```python
from build123d import *

# Parameters (mm, degrees)
EXTRUDE_START                = -12
EXTRUDE_1_DEPTH              = 12
HOLE_WIZARD_M5_1_D           = 4.2
HOLE_WIZARD_M5_1_DEPTH       = 12.4
HOLE_WIZARD_M5_1_CBORE_D     = 5
HOLE_WIZARD_M5_1_CBORE_DEPTH = 10
HOLE_WIZARD_M5_1_TIP         = 1.2618073
HOLE_WIZARD_M5_2_D           = 4.2
HOLE_WIZARD_M5_2_DEPTH       = 12.4
HOLE_WIZARD_M5_2_CBORE_D     = 5
HOLE_WIZARD_M5_2_CBORE_DEPTH = 10
HOLE_WIZARD_M5_2_TIP         = 1.2618073
HOLE_WIZARD_M5_3_D           = 4.2
HOLE_WIZARD_M5_3_DEPTH       = 12.4
HOLE_WIZARD_M5_3_CBORE_D     = 5
HOLE_WIZARD_M5_3_CBORE_DEPTH = 10
HOLE_WIZARD_M5_3_TIP         = 1.2618073
HOLE_WIZARD_M5_4_D           = 4.2
HOLE_WIZARD_M5_4_DEPTH       = 12.4
HOLE_WIZARD_M5_4_CBORE_D     = 5
HOLE_WIZARD_M5_4_CBORE_DEPTH = 10
HOLE_WIZARD_M5_4_TIP         = 1.2618073
HOLE_WIZARD_M5_5_D           = 4.2
HOLE_WIZARD_M5_5_DEPTH       = 12.4
HOLE_WIZARD_M5_5_CBORE_D     = 5
HOLE_WIZARD_M5_5_CBORE_DEPTH = 10
HOLE_WIZARD_M5_5_TIP         = 1.2618073
HOLE_WIZARD_M5_6_D           = 4.2
HOLE_WIZARD_M5_6_DEPTH       = 12.4
HOLE_WIZARD_M5_6_CBORE_D     = 5
HOLE_WIZARD_M5_6_CBORE_DEPTH = 10
HOLE_WIZARD_M5_6_TIP         = 1.2618073
SKETCH_12_R                  = 15.5
CUT_EXTRUDE_1_DEPTH          = 72.996259845
CHAMFER_3_SIZE               = 2
SKETCH_19_R                  = 39.897088004
CUT_EXTRUDE_2_DEPTH          = 15
SKETCH_20_R                  = 21
CUT_EXTRUDE_3_DEPTH          = 16
SKETCH_22_R                  = 19
CUT_EXTRUDE_5_DEPTH          = 2
SKETCH_23_R                  = 30
CUT_EXTRUDE_6_DEPTH          = 4
HOLE_WIZARD_M4_1_D           = 3.3
HOLE_WIZARD_M4_1_DEPTH       = 10.1
HOLE_WIZARD_M4_1_CBORE_D     = 4
HOLE_WIZARD_M4_1_CBORE_DEPTH = 8
HOLE_WIZARD_M4_1_TIP         = 0.991420021
FILLET_1_R                   = 5
FILLET_2_R                   = 2


with BuildPart() as part:
    # 草图1 → 旋转1 (revolve)
    with BuildSketch(Plane.XY, mode=Mode.PRIVATE) as revolve_1_sk:
        Polygon((0, 31.73223769), (-30, 31.73223769), (-30, 11.73223769), (-30, -3.26776231), (-15, -3.26776231), (0, -3.26776231), align=None)
    revolve(revolve_1_sk.sketch.rotate(Axis((0, -1000, 0), (0, 1, 0)), 180), axis=Axis((0, -1000, 0), (0, 1, 0)))

    # 草图2 → 拉伸1 (add)
    with BuildSketch(Plane(origin=(0, 31.73223769, 0), x_dir=(-1, 0, 0), z_dir=(0, 1, 0)).offset(EXTRUDE_START)):
        with BuildLine():
            Line((-33.97114317, 31.160254038), (-19.494897428, 22.802389662))
            ThreePointArc((-19.494897428, 22.802389662), (-25.980762114, 15), (-29.494897428, 5.481881586))
            Line((-29.494897428, 5.481881586), (-43.97114317, 13.839745962))
            Line((-43.97114317, 13.839745962), (-33.97114317, 31.160254038))
        make_face()
        with BuildLine():
            Line((33.97114317, 31.160254038), (43.97114317, 13.839745962))
            Line((43.97114317, 13.839745962), (29.494897428, 5.481881586))
            ThreePointArc((29.494897428, 5.481881586), (25.980762114, 15), (19.494897428, 22.802389662))
            Line((19.494897428, 22.802389662), (33.97114317, 31.160254038))
        make_face()
        with BuildLine():
            Line((10, -28.284271247), (10, -45))
            Line((10, -45), (-10, -45))
            Line((-10, -45), (-10, -28.284271247))
            ThreePointArc((-10, -28.284271247), (0, -30), (10, -28.284271247))
        make_face()
    extrude(amount=EXTRUDE_1_DEPTH)

    # M5 螺纹孔1
    with Locations(Plane(origin=(10, 25.73223769, -39), x_dir=(0, 1, 0), z_dir=(1, 0, 0))):
        with Locations((0, 0)):
            CounterBoreHole(HOLE_WIZARD_M5_1_D / 2, HOLE_WIZARD_M5_1_CBORE_D / 2, HOLE_WIZARD_M5_1_CBORE_DEPTH, depth=HOLE_WIZARD_M5_1_DEPTH)
            with Locations((0, 0, -(HOLE_WIZARD_M5_1_DEPTH + HOLE_WIZARD_M5_1_TIP / 2))):  # 118° drill point
                Cone(0, HOLE_WIZARD_M5_1_D / 2, HOLE_WIZARD_M5_1_TIP, mode=Mode.SUBTRACT)

    # M5 螺纹孔2
    with Locations(Plane.ZY.offset(10)):
        with Locations((-39, 25.73223769)):
            CounterBoreHole(HOLE_WIZARD_M5_2_D / 2, HOLE_WIZARD_M5_2_CBORE_D / 2, HOLE_WIZARD_M5_2_CBORE_DEPTH, depth=HOLE_WIZARD_M5_2_DEPTH)
            with Locations((0, 0, -(HOLE_WIZARD_M5_2_DEPTH + HOLE_WIZARD_M5_2_TIP / 2))):  # 118° drill point
                Cone(0, HOLE_WIZARD_M5_2_D / 2, HOLE_WIZARD_M5_2_TIP, mode=Mode.SUBTRACT)

    # M5 螺纹孔3
    with Locations(Plane(origin=(28.774990748, 25.73223769, 28.160254038), x_dir=(0.866025403784, 0, 0.5), z_dir=(-0.5, 0, 0.866025403784))):
        with Locations((0, 0)):
            CounterBoreHole(HOLE_WIZARD_M5_3_D / 2, HOLE_WIZARD_M5_3_CBORE_D / 2, HOLE_WIZARD_M5_3_CBORE_DEPTH, depth=HOLE_WIZARD_M5_3_DEPTH)
            with Locations((0, 0, -(HOLE_WIZARD_M5_3_DEPTH + HOLE_WIZARD_M5_3_TIP / 2))):  # 118° drill point
                Cone(0, HOLE_WIZARD_M5_3_D / 2, HOLE_WIZARD_M5_3_TIP, mode=Mode.SUBTRACT)

    # M5 螺纹孔4
    with Locations(Plane(origin=(38.774990748, 25.73223769, 10.839745962), x_dir=(-0.866025403784, 0, -0.5), z_dir=(0.5, 0, -0.866025403784))):
        with Locations((0, 0)):
            CounterBoreHole(HOLE_WIZARD_M5_4_D / 2, HOLE_WIZARD_M5_4_CBORE_D / 2, HOLE_WIZARD_M5_4_CBORE_DEPTH, depth=HOLE_WIZARD_M5_4_DEPTH)
            with Locations((0, 0, -(HOLE_WIZARD_M5_4_DEPTH + HOLE_WIZARD_M5_4_TIP / 2))):  # 118° drill point
                Cone(0, HOLE_WIZARD_M5_4_D / 2, HOLE_WIZARD_M5_4_TIP, mode=Mode.SUBTRACT)

    # M5 螺纹孔5
    with Locations(Plane(origin=(-5, 0, -8.660254038), x_dir=(-0.8660254037844396, 1.0079044292037923e-15, 0.4999999999999983), z_dir=(-0.4999999999999983, -1.7457416805546845e-15, -0.8660254037844396))):
        with Locations((39, 25.73223769)):
            CounterBoreHole(HOLE_WIZARD_M5_5_D / 2, HOLE_WIZARD_M5_5_CBORE_D / 2, HOLE_WIZARD_M5_5_CBORE_DEPTH, depth=HOLE_WIZARD_M5_5_DEPTH)
            with Locations((0, 0, -(HOLE_WIZARD_M5_5_DEPTH + HOLE_WIZARD_M5_5_TIP / 2))):  # 118° drill point
                Cone(0, HOLE_WIZARD_M5_5_D / 2, HOLE_WIZARD_M5_5_TIP, mode=Mode.SUBTRACT)

    # M5 螺纹孔6
    with Locations(Plane(origin=(-28.774990748, 25.73223769, 28.160254038), x_dir=(0.866025403784, 0, -0.5), z_dir=(0.5, 0, 0.866025403784))):
        with Locations((0, 0)):
            CounterBoreHole(HOLE_WIZARD_M5_6_D / 2, HOLE_WIZARD_M5_6_CBORE_D / 2, HOLE_WIZARD_M5_6_CBORE_DEPTH, depth=HOLE_WIZARD_M5_6_DEPTH)
            with Locations((0, 0, -(HOLE_WIZARD_M5_6_DEPTH + HOLE_WIZARD_M5_6_TIP / 2))):  # 118° drill point
                Cone(0, HOLE_WIZARD_M5_6_D / 2, HOLE_WIZARD_M5_6_TIP, mode=Mode.SUBTRACT)

    # 草图12 → 切除-拉伸1 (cut, through all)
    with BuildSketch(Plane(origin=(0, 31.73223769, 0), x_dir=(-1, 0, 0), z_dir=(0, 1, 0))):
        Circle(SKETCH_12_R)
    extrude(amount=-CUT_EXTRUDE_1_DEPTH, mode=Mode.SUBTRACT)

    # 倒角3
    chamfer_3_edges = [part.edges().sort_by_distance(p)[0] for p in [
        (-30, -3.26776231, 0),
    ]]
    chamfer(chamfer_3_edges, length=CHAMFER_3_SIZE)

    # 草图19 → 切除-拉伸2 (cut)
    with BuildSketch(Plane.XZ.offset(3.26776231)):
        Circle(SKETCH_19_R)
    extrude(amount=-CUT_EXTRUDE_2_DEPTH, mode=Mode.SUBTRACT)

    # 草图20 → 切除-拉伸3 (cut)
    with BuildSketch(Plane.XZ.offset(-11.73223769)):
        Circle(SKETCH_20_R)
    extrude(amount=-CUT_EXTRUDE_3_DEPTH, mode=Mode.SUBTRACT)

    # 草图22 → 切除-拉伸5 (cut)
    with BuildSketch(Plane.XZ.offset(-27.73223769)):
        Circle(SKETCH_22_R)
    extrude(amount=-CUT_EXTRUDE_5_DEPTH, mode=Mode.SUBTRACT)

    # 草图23 → 切除-拉伸6 (cut)
    with BuildSketch(Plane.XZ.offset(-11.73223769)):
        Circle(SKETCH_23_R)
    extrude(amount=-CUT_EXTRUDE_6_DEPTH, mode=Mode.SUBTRACT)

    # M4 螺纹孔1
    with Locations(Plane(origin=(-12.5, 15.73223769, 21.650635095), x_dir=(-1, 0, 0), z_dir=(0, -1, 0))):
        with Locations((0, 0), (-25, 0), (-37.5, 21.650635095), (-25, 43.30127019), (0, 43.30127019), (12.5, 21.650635095)):
            CounterBoreHole(HOLE_WIZARD_M4_1_D / 2, HOLE_WIZARD_M4_1_CBORE_D / 2, HOLE_WIZARD_M4_1_CBORE_DEPTH, depth=HOLE_WIZARD_M4_1_DEPTH)
            with Locations((0, 0, -(HOLE_WIZARD_M4_1_DEPTH + HOLE_WIZARD_M4_1_TIP / 2))):  # 118° drill point
                Cone(0, HOLE_WIZARD_M4_1_D / 2, HOLE_WIZARD_M4_1_TIP, mode=Mode.SUBTRACT)

    # 圆角1
    fillet_1_edges = [part.edges().sort_by_distance(p)[0] for p in [
        (19.494897428, 25.73223769, 22.802389662),
        (29.494897428, 25.73223769, 5.481881586),
        (10, 25.73223769, -28.284271247),
        (-10, 25.73223769, -28.284271247),
        (-19.494897428, 25.73223769, 22.802389662),
        (-29.494897428, 25.73223769, 5.481881586),
    ]]
    fillet(fillet_1_edges, radius=FILLET_1_R)

    # 圆角2
    fillet_2_edges = [part.edges().sort_by_distance(p)[0] for p in [
        (43.97114317, 25.73223769, 13.839745962),
        (33.97114317, 25.73223769, 31.160254038),
        (-10, 25.73223769, -45),
        (10, 25.73223769, -45),
        (-33.97114317, 25.73223769, 31.160254038),
        (-43.97114317, 25.73223769, 13.839745962),
    ]]
    fillet(fillet_2_edges, radius=FILLET_2_R)


solid = part.part
```
The model under review builds one solid part; all positions refer to its coordinate system, in mm. A direction names the side the tool comes from. Give positions to 0.01 mm unless a question says otherwise; leave off trailing zeros. Write each loop counter-clockwise with the first axis right and the second up, starting at its lowest first coordinate (ties: lowest second). Pieces come first, ordered by that corner, then holes. Notation, with made-up numbers: M 32.25,36 L 70.25,36 A28 ccw 70.25,73 Z; hole C 60,-0.5 d1. An arc over 180 degrees is marked long. Write item = value, one per line. Start each with the question number.
Q1. Mouldability with a two-part tool opening along X and no side actions: class faces 1 (the face through (12.934, 19.676, -19.698)), 2 (the face through (0, 19.732, -36)), 3 (the face through (10, 26, -36)), 4 (the face through (-30.44, 25.82, 5.11)) as released by +X, released by -X, zero draft, split by the parting line, or undercut.
Q2. Clearance check with flat-ended pins moving along their axes: pin 1 (3 mm diameter, centred on y = 24.5, z = 19.5, fed in from -X); pin 2 (2 mm diameter, centred on x = -29, y = 24, fed in from +Z); pin 3 (8 mm diameter, centred on x = 34, z = 21.5, fed in from -Y). State where each tip first meets the part, or that it passes through.
Q3. We need section A-A (z = -39). State the section outline as (x, y) points, plus the area to 3 significant figures.
Q4. Machinability: for faces 5 (the face through (-23, 20, 0)), 6 (the face through (-36.287, 25.648, 9.403)), which of the approach directions +Z, -Z, +X, -X, +Y, -Y give a long, thin tool a straight path to every point of the face, cutting with its end or side? Answer none if there is none.
Q5. For line 1 (Z direction, x = 12, y = 19.5); line 2 (Z direction, x = -13, y = 17.5); line 3 (Y direction, x = 9.5, z = -41), list the stretches that pass through material, from the lowest coordinate up.
Q6. We need section B-B (z = -6). State the section outline as (x, y) points.
Result set:
q1.face_1 = undercut
q1.face_2 = zero draft
q1.face_3 = released by +X
q1.face_4 = released by -X
q2.pin_1 = -41.57
q2.pin_2 = 28.82
q2.pin_3 = 19.73
q3.outline = M -10,19.73 L 10,19.73 L 10,23.23 L -10,23.23 Z; M -10,28.23 L 10,28.23 L 10,31.73 L -10,31.73 Z
q3.area = 140 mm2
q4.face_5 = -Y
q4.face_6 = -Z, -X, +Y, -Y
q5.line_1 = -27.5 to -23.59, -19.71 to -17.23, 17.23 to 19.71, 23.59 to 27.5
q5.line_2 = -27.04 to -23.59, -19.71 to -16.49, 16.49 to 19.71, 23.59 to 27.04
q5.line_3 = 19.73 to 24.23, 27.23 to 31.73
q6.outline = M -29.39,15.73 L -20.12,15.73 L -20.12,27.73 L -18.03,27.73 L -18.03,29.73 L -14.29,29.73 L -14.29,31.73 L -29.39,31.73 Z; M 14.29,29.73 L 18.03,29.73 L 18.03,27.73 L 20.12,27.73 L 20.12,15.73 L 29.39,15.73 L 29.39,31.73 L 14.29,31.73 Z
